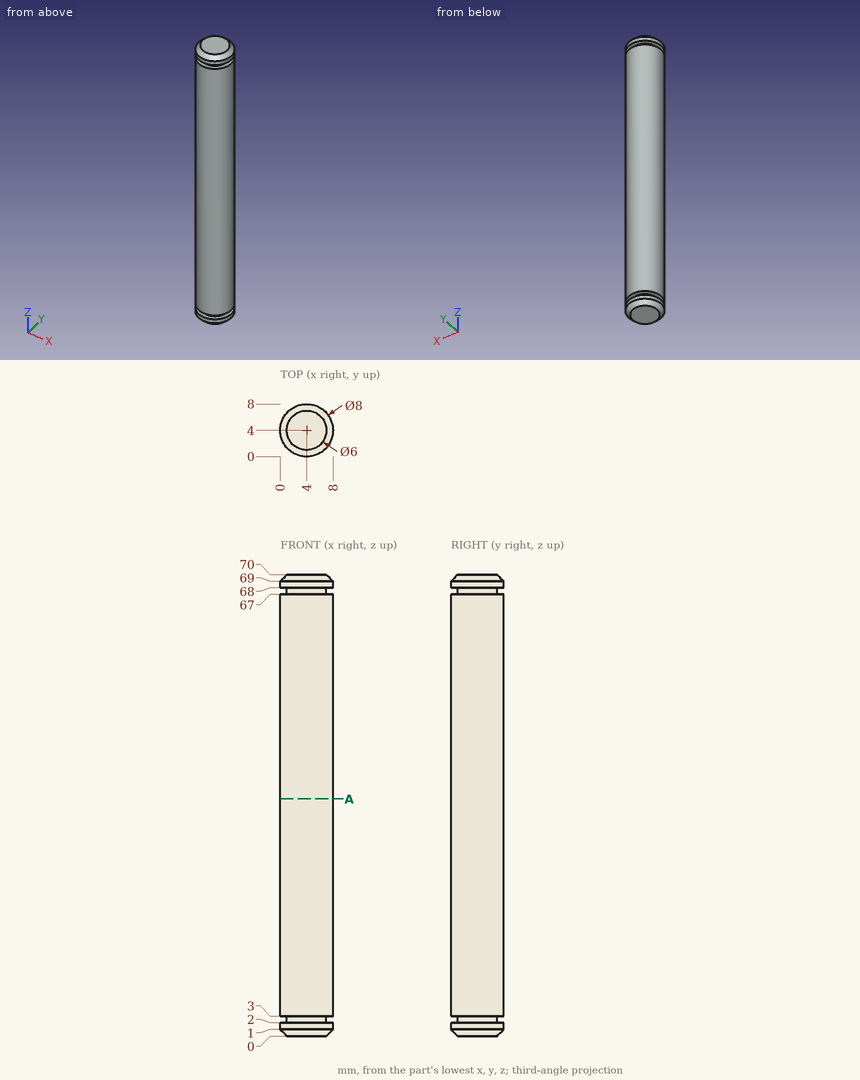
Input: dimensioned drawing with shaded views. Units: mm. Origin: part minimum x, y, z. Coordinates: 2 decimals unless noted, no trailing zeros. Write each loop counter-clockwise with the first axis right and the second up, starting at its lowest first coordinate (ties: lowest second). Pieces come first, ordered by that corner, then holes. Notation, with made-up numbers: (-26, 43) -> (-21, 43) arc R10 ccw to (-21, 58) -> close; hole circle Ø3 at (-33, -4.5). An arc over 180 degrees is marked (long way). Return JSON: item names as keys, results as strings. Group by question number.
1) Ray query, line 1 along Z through (x, y) = (0.75, 1.75); line 2 along Z through (x, y) = (6.25, 7); line 3 along Y through (x, z) = (3.75, 22.5). Return the intervals inside material, ascending.
2) Contact query for flat-ended pins moving along their axis: P1, Ø1, axis at y = 5.5, z = 11.5, coming from the -X side; P2, Ø2, axis at y = 1, z = 31, coming from the -X side. Output: stop coordinate, or through.
3) Section query A-A, the plane z = 36. Return loops of the section in (x, y), plus the area to 3 significant figures.
From the geometry:
{
 "1": {"line 1": "0.95 to 2, 3 to 67, 68 to 69.05", "line 2": "0.75 to 2, 3 to 67, 68 to 69.25", "line 3": "0.01 to 7.99"},
 "2": {"P1": "x = 0.13", "P2": "x = 0.54"},
 "3": {"outline": "circle Ø8 at (4, 4)", "area": "50.3 mm²"}
}
